For this review, take the finished solid that the model builds, in its own axes (mm). Face numbers are marked on the shaded views. A direction names the side the tool comes from. Give positions to 0.01 mm unless a question says otherwise; leave off trailing zeros. Write each loop counter-clockwise with the first axis right and the second up, starting at its lowest first coordinate (ties: lowest second). Pieces come first, ordered by that corner, then holes. Notation, with made-up numbers: M 89,54 L 93,54 A30 cw 93,84 Z; hole C 36.25,43.25 d7. An arc over 180 degrees is marked long. One line per item, written item: value. Start each with the question number.
Item 1: Tool access review of the marked faces 1 and 2: name each direction out of +Z, -Z, +X, -X, +Y, -Y from which nothing blocks a thin tool from reaching the whole face with its end or side.
Item 2: Consider section A-A, the plane x = -166. Write out the cut boundary in (y, z).
Item 3: Consider section C-C, the plane z = 44. Write out the cut boundary in (x, y), and give its area (3 significant figures).
Item 4: Consider section B-B, the plane y = -348.5. Write out the cut boundary in (x, z), and give its area (3 significant figures).
Item 5: To check wall thickness, follow probe 1 along X at (y, z) = (-139.5, 15.5); probe 2 along Y at (x, z) = (-480, 115). State the ranges of each line that lie inside material, in increasing order.
Item 6: Mouldability with a two-part tool opening along X and no side actions: class the marked faces 3, 4 and 5 as released by +X, released by -X, zero draft, split by the parting line, or undercut.
Autodesk Inventor part; units mm, degrees
ref_plane "YZ Plane" through (0, 0, 0) normal (1, 0, 0) x (0, 1, 0)
ref_plane "XZ Plane" through (0, 0, 0) normal (0, 1, 0) x (-1, 0, 0)
ref_plane "XY Plane" through (0, 0, 0) normal (0, 0, 1) x (1, 0, 0)
sketch "Esquisse1" plane through (0, 0, 0) normal (0, 0, 1) x (1, 0, 0)
  line L0 (-745.614, 899.1228) -> (754.386, 899.1228)
  line L1 (754.386, 899.1228) -> (754.386, -1000.8772)
  line L2 (754.386, -1000.8772) -> (-745.614, -1000.8772)
  line L3 (-745.614, -1000.8772) -> (-745.614, 899.1228)
  point P0 (0, 0)
  dimension "d0" = 1500
  dimension "d1" = 1900
extrude "Extrusion1" add sketch "Esquisse1" along normal blind 200
sketch "Esquisse2" plane through (0, 0, 200) normal (0, 0, 1) x (1, 0, 0)
  line L0 (-565.614, 819.1228) -> (-55.614, 819.1228)
  line L1 (-55.614, 819.1228) -> (-55.614, -800.8772)
  line L2 (-55.614, -800.8772) -> (-565.614, -800.8772)
  line L3 (-565.614, -800.8772) -> (-565.614, 819.1228)
  line L4 (64.386, 819.1228) -> (574.386, 819.1228)
  line L5 (574.386, 819.1228) -> (574.386, -800.8772)
  line L6 (574.386, -800.8772) -> (64.386, -800.8772)
  line L7 (64.386, -800.8772) -> (64.386, 819.1228)
  line L8 (-745.614, 899.1228) -> (-745.614, -1000.8772)
  line L9 (754.386, -1000.8772) -> (754.386, 899.1228)
  line L10 (-745.614, -1000.8772) -> (754.386, -1000.8772)
  point P0 (0, 0)
  dimension "d4" = 510
  dimension "d5" = 510
  dimension "d6" = 1620
  dimension "d7" = 1620
  dimension "d8" = 180
  dimension "d9" = 180
  dimension "d10" = 200
extrude "Extrusion2" cut sketch "Esquisse2" against normal blind 200
properties part number "Fenetre-Bords" material "Plastique ABS"
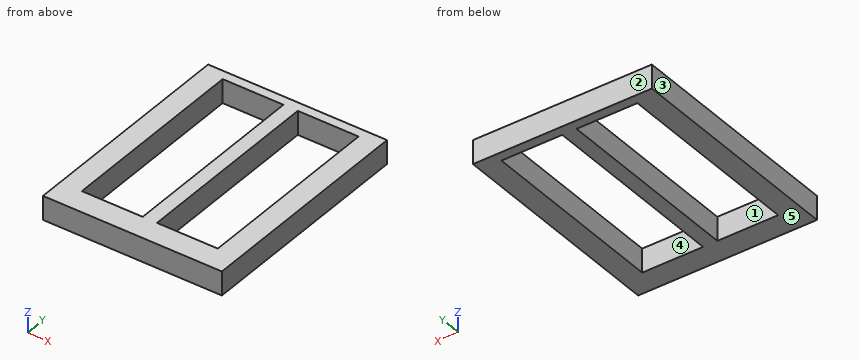
Model answer:
1. face 1: +Z, -Z
1. face 2: +Z, -Z, +X, -X, +Y
2. outline: M -1000.88,0 L -800.88,0 L -800.88,200 L -1000.88,200 Z; M 819.12,0 L 899.12,0 L 899.12,200 L 819.12,200 Z
3. outline: M -745.61,-1000.88 L 754.39,-1000.88 L 754.39,899.12 L -745.61,899.12 Z; hole M -565.61,-800.88 L -55.61,-800.88 L -55.61,819.12 L -565.61,819.12 Z; hole M 64.39,-800.88 L 574.39,-800.88 L 574.39,819.12 L 64.39,819.12 Z
3. area: 1,200,000 mm2
4. outline: M -745.61,0 L -565.61,0 L -565.61,200 L -745.61,200 Z; M -55.61,0 L 64.39,0 L 64.39,200 L -55.61,200 Z; M 574.39,0 L 754.39,0 L 754.39,200 L 574.39,200 Z
4. area: 96,000 mm2
5. probe 1: x = -745.61 to -565.61, -55.61 to 64.39, 574.39 to 754.39
5. probe 2: y = -1000.88 to -800.88, 819.12 to 899.12
6. face 3: released by -X
6. face 4: undercut
6. face 5: zero draft
